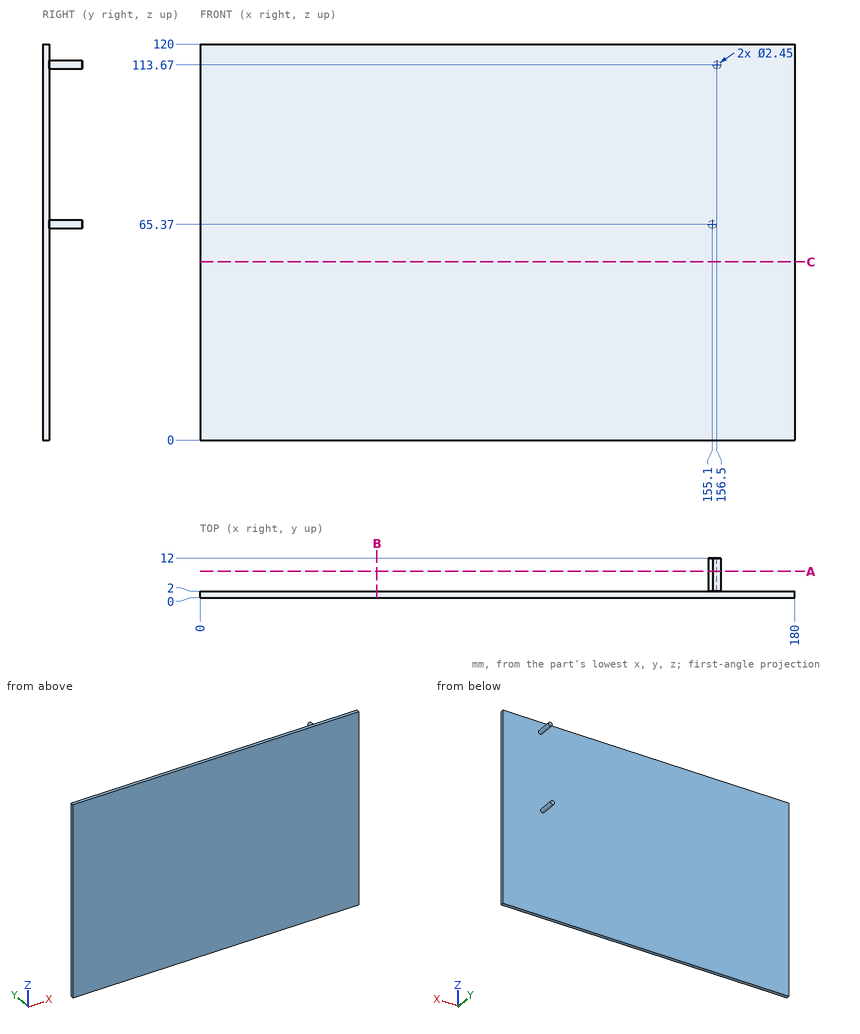
Design review of the part shown in the three views and the two pictorial views. Dimensions are in mm from the part's minimum x, y and z. Round coordinates to 2 decimals unless told otherwise and drop trailing zeros. Write each loop counter-clockwise with the first axis right and the second up, starting at its lowest first coordinate (ties: lowest second). Pieces come first, ordered by that corner, then holes. Notation, with made-up numbers: (-39.5, -40) -> (-23.5, -40) arc R21 ccw to (-23.5, -8) -> close; hole circle Ø8 at (55.5, 69). An arc over 180 degrees is marked (long way). Use one line per item in the form item = value.
1) Clearance check with a flat-ended pin moving along its axis: pin 1 (12 mm diameter, centred on x = 34.5, z = 71, fed in from +Y). State where the tip first meets the part, or that it passes through.
Found:
pin_1 = 2
2) To check wall thickness, follow L1, parallel to Y at x = 61, z = 62. State the ranges of the line that lie inside material, in increasing order. Write a range as from..to.
Found:
L1 = 0..2
3) Take a section at A-A, the plane y = 8. Write out the cut boundary in (x, z) (3 decimals), and give its area (3 significant figures).
Found:
outline = circle Ø2.45 at (155.1, 65.37); circle Ø2.45 at (156.5, 113.67)
area = 9.43 mm2
4) Take a section at C-C, the plane z = 54. Write out the cut boundary in (x, y).
Found:
outline = (0, 0) -> (180, 0) -> (180, 2) -> (0, 2) -> close
5) Take a section at B-B, the plane x = 53.5. Write out the cut boundary in (y, z).
Found:
outline = (0, 0) -> (2, 0) -> (2, 120) -> (0, 120) -> close
